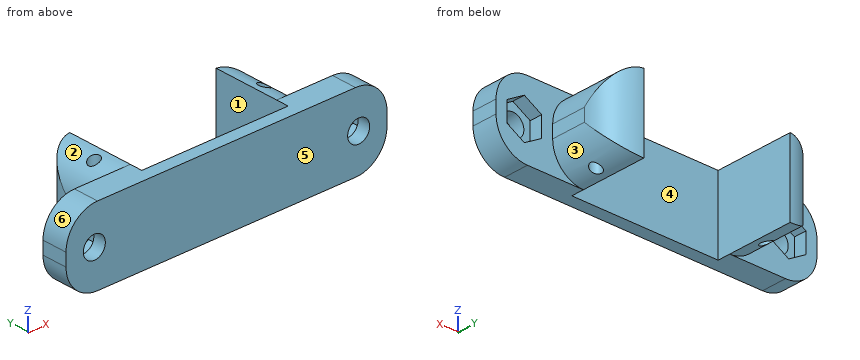
```python
from build123d import *

# Parameters (mm, degrees)
F0_R        = 0.875
F1_DEPTH    = 12
F2_R        = 1.75
F3_DEPTH    = 25
F4_DEPTH    = 2
F5_T1_DEPTH = 36.9921862789
F5_T3_DEPTH = 29
F5_T5_DEPTH = 22.9960931395


# Not quite as in the source:
# - a fillet or chamfer that OpenCascade refuses, or shapes differently, is made with other operations: its cross-section is extruded or revolved along the edge and cut away or added


with BuildPart() as f1:
    # F0 (on Top) → F1 (new body)
    with BuildSketch(Plane.XY):
        Polygon((-11.625, 7.25), (-16.5, 7.25), (-16.5, -3.25), (-16.5, -5.25), (-11.625, -5.25), align=None)
        with Locations((-13.5, 1)):
            Circle(F0_R, mode=Mode.SUBTRACT)
        Polygon((-16.5, -5.25), (-16.5, -3.25), (-25.5, -3.25), (-25.5, -7.25), (-16.5, -7.25), align=None)
        Polygon((11.625, -5.25), (-11.625, -5.25), (-16.5, -5.25), (-16.5, -7.25), (16.5, -7.25), (16.5, -5.25), align=None)
        Polygon((25.5, -3.25), (16.5, -3.25), (16.5, -5.25), (16.5, -7.25), (25.5, -7.25), align=None)
        Polygon((16.5, 7.25), (11.625, 7.25), (11.625, -5.25), (16.5, -5.25), (16.5, -3.25), align=None)
        with Locations((13.5, 1)):
            Circle(F0_R, mode=Mode.SUBTRACT)
    extrude(amount=F1_DEPTH)

    # F2 (on face) → F3 (cut)
    with BuildSketch(Plane(origin=(0, -3.25, 0), x_dir=(-1, 0, 0), z_dir=(0, 1, 0))):
        with Locations((-21, 6)):
            Circle(F2_R)
        with Locations((21, 6)):
            Circle(F2_R)
    extrude(amount=-F3_DEPTH, mode=Mode.SUBTRACT)

    # F2 (on face) → F4 (cut)
    with BuildSketch(Plane(origin=(0, -3.25, 0), x_dir=(-1, 0, 0), z_dir=(0, 1, 0))):
        Polygon((-23.75, 7.5877132403), (-23.75, 4.4122867597), (-21, 2.8245735195), (-18.25, 4.4122867597), (-18.25, 7.5877132403), (-21, 9.1754264805), align=None)
        with Locations((-21, 6)):
            Circle(F2_R, mode=Mode.SUBTRACT)
        Polygon((23.75, 4.4122867597), (23.75, 7.5877132403), (21, 9.1754264805), (18.25, 7.5877132403), (18.25, 4.4122867597), (21, 2.8245735195), align=None)
        with Locations((21, 6)):
            Circle(F2_R, mode=Mode.SUBTRACT)
    extrude(amount=-F4_DEPTH, mode=Mode.SUBTRACT)

    # F5: fillet of radius 5 on 10 edges, made by hand

    # F5_s2 → F5_t1 (cut)
    with BuildSketch(Plane.XY.offset(-12.4960931395)):
        with BuildLine():
            ThreePointArc((-11.625, 7.25), (-15.0794552658, 5.7426227552), (-16.5, 2.2515627442))
            Line((-16.5, 2.2515627442), (-16.5, 7.25))
            Line((-16.5, 7.25), (-11.625, 7.25))
        make_face()
        with BuildLine():
            ThreePointArc((16.5, 2.2515627442), (15.0794552658, 5.7426227552), (11.625, 7.25))
            Line((11.625, 7.25), (16.5, 7.25))
            Line((16.5, 7.25), (16.5, 2.2515627442))
        make_face()
    extrude(amount=F5_T1_DEPTH, mode=Mode.SUBTRACT)

    # F5_s4 → F5_t3 (cut)
    with BuildSketch(Plane.XZ.offset(-9.25)):
        with BuildLine():
            ThreePointArc((20.5, 12), (24.0355339059, 10.5355339059), (25.5, 7))
            Line((25.5, 7), (25.5, 12))
            Line((25.5, 12), (20.5, 12))
        make_face()
        with BuildLine():
            ThreePointArc((20.5, 0), (24.0355339059, 1.4644660941), (25.5, 5))
            Line((25.5, 5), (25.5, 0))
            Line((25.5, 0), (20.5, 0))
        make_face()
        with BuildLine():
            ThreePointArc((-20.5, 0), (-24.0355339059, 1.4644660941), (-25.5, 5))
            Line((-25.5, 5), (-25.5, 0))
            Line((-25.5, 0), (-20.5, 0))
        make_face()
        with BuildLine():
            ThreePointArc((-20.5, 12), (-24.0355339059, 10.5355339059), (-25.5, 7))
            Line((-25.5, 7), (-25.5, 12))
            Line((-25.5, 12), (-20.5, 12))
        make_face()
    extrude(amount=F5_T3_DEPTH, mode=Mode.SUBTRACT)

    # F5_s6 → F5_t5 (cut)
    with BuildSketch(Plane.XZ.offset(-19.7460931395)):
        with BuildLine():
            ThreePointArc((11.625, 0), (15.0794552658, 1.5073772448), (16.5, 4.9984372558))
            Line((16.5, 4.9984372558), (16.5, 0))
            Line((16.5, 0), (11.625, 0))
        make_face()
        with BuildLine():
            ThreePointArc((11.625, 12), (15.0794552658, 10.4926227552), (16.5, 7.0015627442))
            Line((16.5, 7.0015627442), (16.5, 12))
            Line((16.5, 12), (11.625, 12))
        make_face()
        with BuildLine():
            ThreePointArc((-16.5, 7.0015627442), (-15.0794552658, 10.4926227552), (-11.625, 12))
            Line((-11.625, 12), (-16.5, 12))
            Line((-16.5, 12), (-16.5, 7.0015627442))
        make_face()
        with BuildLine():
            ThreePointArc((-16.5, 4.9984372558), (-15.0794552658, 1.5073772448), (-11.625, 0))
            Line((-11.625, 0), (-16.5, 0))
            Line((-16.5, 0), (-16.5, 4.9984372558))
        make_face()
    extrude(amount=F5_T5_DEPTH, mode=Mode.SUBTRACT)


solid = f1.part
```
Check sheet for the modelled part. Datum: model origin and axes. Units: mm. Face numbers are marked on the shaded views. A direction names the side the tool comes from. Coordinates: 2 decimals unless noted, no trailing zeros. Loops run counter-clockwise (first coordinate to the right, second up) from the corner with the lowest first, then second, coordinate; pieces in that order, holes last.
1) Sectioned sample at D-D (x = -13.5). Record the boundary of the cut face in (y, z) (3 decimals), and give its area (3 significant figures).
2) Sectioned sample at C-C (y = -1). Record the boundary of the cut face in (x, z) (3 decimals), and give its area (3 significant figures).
3) Gauge pin test, flat ends, axial feed: pin 1 (1.4 mm diameter, centred on x = 13.5, y = 1, fed in from +Z); pin 2 (4.5 mm diameter, centred on x = 20.5, z = 7.5, fed in from +Y); pin 3 (3 mm diameter, centred on x = -13.5, y = 1, fed in from -Z); pin 4 (4 mm diameter, centred on x = 21, z = 6, fed in from +Y). Record the tip position at first contact, or that the pin passes through.
4) Access from +Z, -Z, +X, -X, +Y, -Y to the whole of each face (thin tool, end or side, straight path). Record for the marked faces 1, 2 and 3.
5) Release check for a two-part mould opening along X. For the marked faces 4, 5 and 6 record: released by +X, released by -X, zero draft, split by the parting line, or undercut.
6) Sectioned sample at B-B (y = -4.75). Record the boundary of the cut face in (x, z) (3 decimals), and give its area (3 significant figures).
7) Material ranges on probe 1 along X at (y, z) = (1, 5.25) (3 decimals); probe 2 along X at (y, z) = (1, 8) (3 decimals); probe 3 along Y at (x, z) = (0, 9), recorded low to high.
8) Sectioned sample at A-A (z = 6). Count the separate pieces of the cut face and the enclosed holes in it, and give its area (3 significant figures).
Check sheet entries:
1. outline: (-7.25, 0) - (-3.25, 0) - (-3.25, 0.416) - (0.125, 0.416) - (0.125, 11.584) - (-3.25, 11.584) - (-3.25, 12) - (-7.25, 12) - close; (1.875, 0.416) - (6.834, 0.416) - (6.834, 11.584) - (1.875, 11.584) - close
1. area: 141 mm2
2. outline: (-16.5, 4.998) arc R5 ccw to (-11.625, 0) - (-11.625, 12) arc R5 ccw to (-16.5, 7.002) - close; (11.625, 0) arc R5 ccw to (16.5, 4.998) - (16.5, 7.002) arc R5 ccw to (11.625, 12) - close
2. area: 95.6 mm2
3. pin 1: passes through
3. pin 2: stops at y = -3.25
3. pin 3: stops at z = 0.02
3. pin 4: stops at y = -5.25
4. face 1: +Z, -Z, +Y
4. face 2: +Z, -X, +Y
4. face 3: -Z, +X, +Y
5. face 4: undercut
5. face 5: zero draft
5. face 6: released by -X
6. outline: (-25.5, 5) arc R5 ccw to (-20.5, 0) - (-11.625, 0) - (-11.625, 12) - (-20.5, 12) arc R5 ccw to (-25.5, 7) - close; (11.625, 0) - (20.5, 0) arc R5 ccw to (25.5, 5) - (25.5, 7) arc R5 ccw to (20.5, 12) - (11.625, 12) - close; hole (-23.75, 4.412) - (-21, 2.825) - (-18.25, 4.412) - (-18.25, 7.588) - (-21, 9.175) - (-23.75, 7.588) - close; hole (18.25, 4.412) - (21, 2.825) - (23.75, 4.412) - (23.75, 7.588) - (21, 9.175) - (18.25, 7.588) - close
6. area: 259 mm2
7. probe 1: x = -16.5 to -14.375, -12.625 to -11.625, 11.625 to 12.625, 14.375 to 16.5
7. probe 2: x = -16.399 to -14.375, -12.625 to -11.625, 11.625 to 12.625, 14.375 to 16.399
7. probe 3: y = -7.25 to -5.25
8. separate pieces: 3
8. enclosed holes: 2
8. area: 208 mm2
